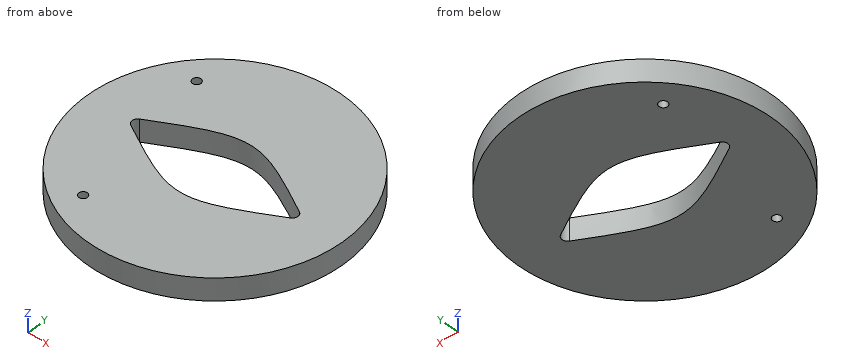
from build123d import *

# Parameters (mm, degrees)
F0_R     = 115
F1_DEPTH = 20
F2_R     = 5
F3_R     = 3.7625
F4_DEPTH = 25


with BuildPart() as f1:
    # F0 (on Top) → F1 (new body)
    with BuildSketch(Plane.XY):
        Circle(F0_R)
        with BuildLine():
            add(Edge.make_bspline(
                [(-80, 0), (0, -45.502603054), (0, -45.502603054), (80, 0)],
                knots=[0, 0, 0, 0, 160, 160, 160, 160], degree=3))
            add(Edge.make_bspline(
                [(-80, 0), (0, 45.502603054), (0, 45.502603054), (80, 0)],
                knots=[0, 0, 0, 0, 160, 160, 160, 160], degree=3))
        make_face(mode=Mode.SUBTRACT)
    extrude(amount=F1_DEPTH)

    # F2
    f2_edges = [f1.edges().sort_by_distance(p)[0] for p in [
        (-80, 0, 10),
        (80, 0, 10),
    ]]
    fillet(f2_edges, radius=F2_R)

    # F3 (on Top) → F4 (cut)
    with BuildSketch(Plane.XY):
        with Locations((-70.8591109885, 59.457853896)):
            Circle(F3_R)
        with Locations((-46.25, -80.1073498501)):
            Circle(F3_R)
    extrude(amount=F4_DEPTH, mode=Mode.SUBTRACT)


solid = f1.part
For this review, take the finished solid that the model builds, in its own axes (mm). Give positions to 0.01 mm unless a question says otherwise; leave off trailing zeros. Loops run counter-clockwise (first coordinate to the right, second up) from the corner with the lowest first, then second, coordinate; pieces in that order, holes last. Notation, with made-up numbers: (71.25, 84) - (87.25, 84) arc R27 ccw to (87.25, 100) - close; hole circle Ø6 at (10, -3). An arc over 180 degrees is marked (long way). Write each question's results on one line, items separated by ' | '.
(1) Take a section at A-A (x = -46.25). State how many separate pieces and enclosed holes the cut face has, then the cut area to 3 significant figures.
Conclusion:
separate pieces: 3 | enclosed holes: 0 | area: 3,310 mm^2
(2) For pin 1 Ø4 at (y, z) = (-32, 6) entering from -X; pin 2 Ø1 at (y, z) = (-70.5, 10) entering from -X; pin 3 Ø6 at (y, z) = (-73, 13.5) entering from +X; pin 4 Ø8 at (x, y) = (59, -17) entering from -Z, all flat-tipped, find the tip position at first contact; note any pin that passes through.
Conclusion:
pin 1: x = -111.02 | pin 2: x = -91.24 | pin 3: x = 91.24 | pin 4: z = 0
(3) For line 1 along Y through (x, z) = (-46.25, 14); line 2 along Y through (x, z) = (-42, 17.75); line 3 along X through (y, z) = (10.5, 18), list the stretches that pass through material, from the lowest coordinate up.
Conclusion:
line 1: -105.29 to -83.87, -76.34 to -18.79, 18.79 to 105.29 | line 2: -107.06 to -20.99, 20.99 to 107.06 | line 3: -114.52 to -61.44, 61.44 to 114.52
(4) Take a section at B-B (y = -56.5). Give the boundary of the cut face in (x, z), then the cut area to 3 significant figures.
Conclusion:
outline: (-100.16, 0) - (100.16, 0) - (100.16, 20) - (-100.16, 20) - close | area: 4,010 mm^2
(5) Take a section at D-D (x = 90.5). Give the boundary of the cut face in (y, z).
Conclusion:
outline: (-70.96, 0) - (70.96, 0) - (70.96, 20) - (-70.96, 20) - close
